The figure shows three views and two pictorial views of one solid part (mm, origin at its lowest corner). Answer the questions. Round coordinates to 2 decimals unless told otherwise and drop trailing zeros. Write each loop counter-clockwise with the first axis right and the second up, starting at its lowest first coordinate (ties: lowest second). Pieces come first, ordered by that corner, then holes.
Item 1: This flat-tipped pin is pushed along its axis until it touches: pin 1 (8 mm diameter, centred on x = 955, y = 564, fed in from -Z). Where does it stop, or does it pass through?
Item 2: Find section A-A on z = 189.5. Give the vertices of the cut face in (x, y).
Item 3: Find section C-C on x = 699. Give the vertices of the cut face in (y, z), then the cut area to 3 significant figures.
Item 4: Find section B-B on y = 449.5. Give the vertices of the cut face in (x, z), then the cut area to 3 significant figures.
Item 5: For a pull along Z with two mould halves and no side action, classify the marked faces 1 and 2 as +Z half, -Z half, draft (parallel to the pull), parting line (faces both ways), or undercut.
Item 6: Find the intervals of material crossed by probe 1 along Z at (x, y) = (588.5, 821); probe 2 along Z at (x, y) = (1445, 251.5), in increasing order.
Item 7: Find section D-D on x = 1380. Give the vertices of the cut face in (y, z).
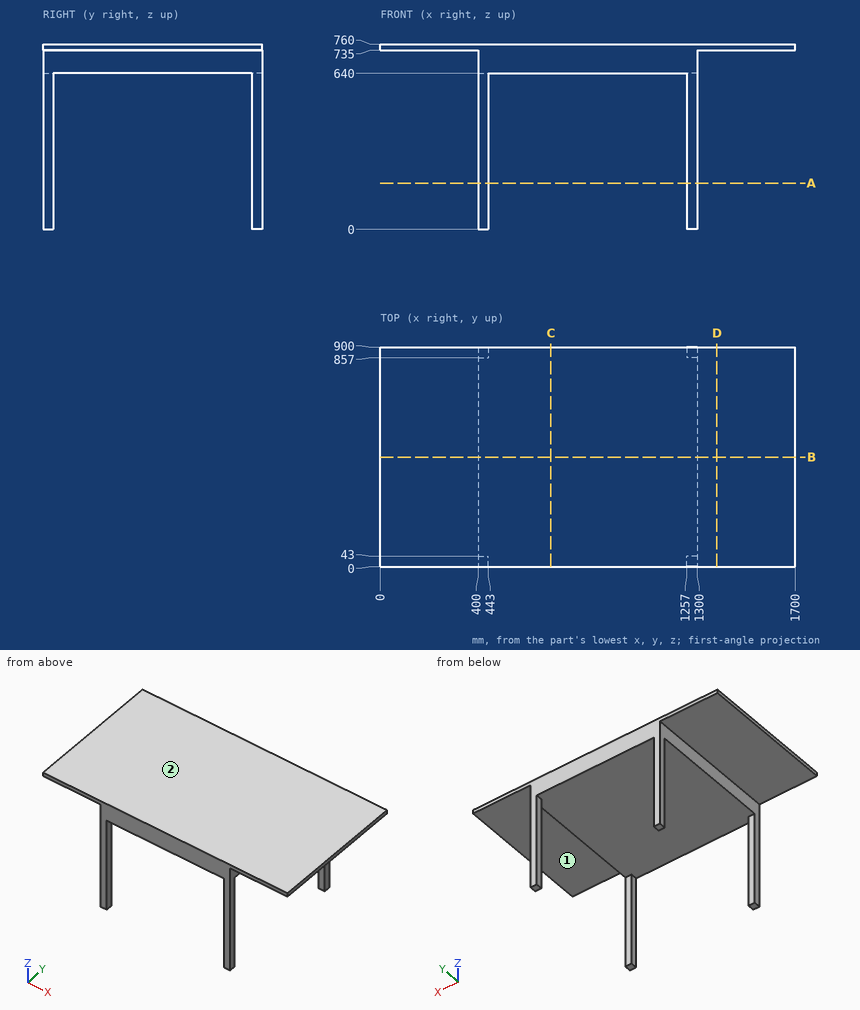
Check values:
1. pin 1: stops at z = 640
2. outline: (400, 0) - (443, 0) - (443, 43) - (400, 43) - close; (400, 857) - (443, 857) - (443, 900) - (400, 900) - close; (1257, 0) - (1300, 0) - (1300, 43) - (1257, 43) - close; (1257, 857) - (1300, 857) - (1300, 900) - (1257, 900) - close
3. outline: (0, 640) - (900, 640) - (900, 760) - (0, 760) - close
3. area: 108,000 mm2
4. outline: (0, 735) - (400, 735) - (400, 640) - (1300, 640) - (1300, 735) - (1700, 735) - (1700, 760) - (0, 760) - close
4. area: 128,000 mm2
5. face 1: -Z half
5. face 2: +Z half
6. probe 1: z = 640 to 760
6. probe 2: z = 735 to 760
7. outline: (0, 735) - (900, 735) - (900, 760) - (0, 760) - close
